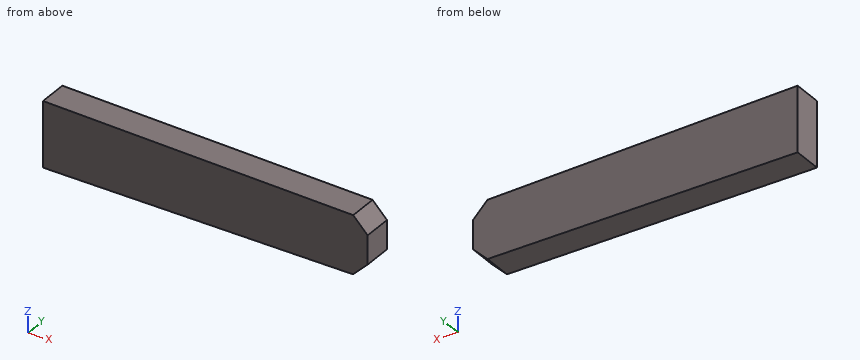
from build123d import *

# Parameters (mm, degrees)
BOSS_EXTRUDE1_DEPTH   = 4
CHAMFER2_SIZE2        = 2
CHAMFER2_SIZE         = 2.023746482
CHAMFER2_EDGE_2_SIZE2 = 2
CHAMFER2_EDGE_2_SIZE  = 2.023746482


with BuildPart() as part:
    # Sketch2 → Boss-Extrude1 (new body)
    with BuildSketch(Plane(origin=(0, 0, 0), x_dir=(1, 0, 0), z_dir=(0, 1, 0))):
        Polygon((0, 9.05), (45, 8.525), (45, 0.525), (0, 0), align=None)
    extrude(amount=BOSS_EXTRUDE1_DEPTH)

    # Chamfer2
    chamfer2_edges = [part.edges().sort_by_distance(p)[0] for p in [
        (45, 2, -8.525),
    ]]
    chamfer(chamfer2_edges, length=CHAMFER2_SIZE, length2=CHAMFER2_SIZE2)

    # Chamfer2 edge 2
    chamfer2_edge_2_edges = [part.edges().sort_by_distance(p)[0] for p in [
        (45, 2, -0.525),
    ]]
    chamfer(chamfer2_edge_2_edges, length=CHAMFER2_EDGE_2_SIZE, length2=CHAMFER2_EDGE_2_SIZE2)


solid = part.part
Model file for the job. Use its own axes, mm. Give positions to 0.01 mm unless a question says otherwise; leave off trailing zeros. Write each loop counter-clockwise with the first axis right and the second up, starting at its lowest first coordinate (ties: lowest second). Pieces come first, ordered by that corner, then holes. Notation, with made-up numbers: M 62.5,-17 L 66.5,-17 A21 ccw 66.5,-6 Z; hole C 75.25,28 d1. An arc over 180 degrees is marked long. One line per item, written item: value. Start each with the question number.
Q1. Saw through at C-C, the plane z = -1.25. Write the cut outline in (x, y), plus the area to 3 significant figures.
Q2. Probe probe 1 along Z at (x, y) = (33, 2.95) (3 decimals); probe 2 along Z at (x, y) = (2, 3.85); probe 3 along X at (y, z) = (2, -1). List the from-to ranges inside material, lowest first. Write a range as [from, to].
Q3. Saw through at B-B, the plane x = 12. Write the cut outline in (y, z).
Q4. Drop a flat-ended pin along its axis: pin 1 Ø1 at (x, y) = (39.5, 2.5) entering from +Z (3 decimals). Give the stop position or say it passes through.
Q5. Saw through at A-A, the plane y = 0.4. Write the cut outline in (x, z) (3 decimals).
Output values:
1. outline: M 0,0 L 43.73,0 L 43.73,4 L 0,4 Z
1. area: 175 mm²
2. probe 1: z = [-8.665, -0.385]
2. probe 2: z = [-9.03, -0.02]
2. probe 3: x = [0, 43.49]
3. outline: M 0,-8.91 L 4,-8.91 L 4,-0.14 L 0,-0.14 Z
4. pin 1: stops at z = -0.455
5. outline: M 0,-9.05 L 42.976,-8.549 L 45,-6.525 L 45,-2.549 L 43,-0.502 L 0,0 Z
